Study the drawing (mm; zero at the part's minimum x, y, z) and answer. A direction names the side the tool comes from. Round coordinates to 2 decimals unless told otherwise and drop trailing zeros. Write each loop counter-clockwise with the first axis right and the second up, starting at its lowest first coordinate (ties: lowest second). Pieces come first, ordered by that corner, then holes.
(1) Each of these flat-tipped pins is pushed along its axis until it touches: pin 1 Ø4 at (y, z) = (7.5, 4.5) entering from +X; pin 2 Ø2.5 at (x, y) = (31, 4) entering from +Z; pin 3 Ø1.2 at (y, z) = (7, 20.5) entering from -X. Where does it stop, or does it pass through?
(2) A cutting plane is placed at A-A, the plane x = 11. Give the vertices of the cut face in (y, z), and give its area (3 significant figures).
(3) A cutting plane is placed at D-D, the plane y = 6.1. Give the vertices of the cut face in (x, z).
(4) Find the intervals of material crossed by probe 1 along Z at (x, y) = (8.5, 4.5); probe 2 along Z at (x, y) = (31, 7.5); probe 3 along X at (y, z) = (9.25, 2.5), in increasing order.
(5) For the marked faces 1, 2 and 3, determine the directions among +Z, -Z, +X, -X, +Y, -Y from which every point of the face is accessible in a straight line to the end or side of a thin tool.
(6) A cutting plane is placed at B-B, the plane y = 2. Give the vertices of the cut face in (x, z).
(7) A cutting plane is placed at C-C, the plane z = 2.5. Give the vertices of the cut face in (x, y), and give its area (3 significant figures).
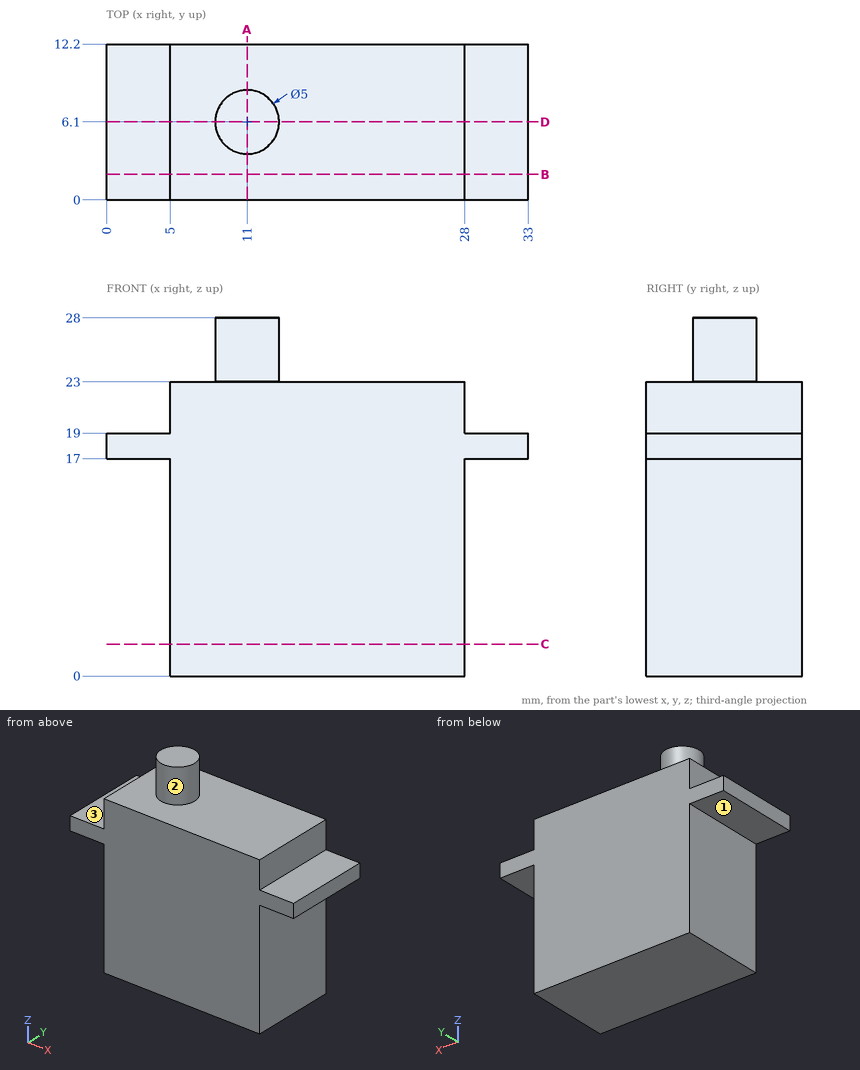
Solutions:
1. pin 1: stops at x = 28
1. pin 2: stops at z = 19
1. pin 3: stops at x = 5
2. outline: (0, 0) - (12.2, 0) - (12.2, 23) - (8.6, 23) - (8.6, 28) - (3.6, 28) - (3.6, 23) - (0, 23) - close
2. area: 306 mm2
3. outline: (0, 17) - (5, 17) - (5, 0) - (28, 0) - (28, 17) - (33, 17) - (33, 19) - (28, 19) - (28, 23) - (13.5, 23) - (13.5, 28) - (8.5, 28) - (8.5, 23) - (5, 23) - (5, 19) - (0, 19) - close
4. probe 1: z = 0 to 23
4. probe 2: z = 17 to 19
4. probe 3: x = 5 to 28
5. face 1: -Z, -X, +Y, -Y
5. face 2: +Z
5. face 3: +Z, -X, +Y, -Y
6. outline: (0, 17) - (5, 17) - (5, 0) - (28, 0) - (28, 17) - (33, 17) - (33, 19) - (28, 19) - (28, 23) - (5, 23) - (5, 19) - (0, 19) - close
7. outline: (5, 0) - (28, 0) - (28, 12.2) - (5, 12.2) - close
7. area: 281 mm2
